CAD build for the part. Positions are in the model's coordinates, mm. Face numbers are marked on the shaded views. A direction names the side the tool comes from. Round coordinates to 2 decimals unless told otherwise and drop trailing zeros. Order: outer loops, then holes, each group sorted by start corner. A loop starts at its lowest first (then second) coordinate and runs counter-clockwise, first axis right, second up. Notation, with made-up numbers: (53, 18.5) -> (70, 18.5) arc R10 ccw to (70, 34.5) -> close; hole circle Ø10 at (37, 72.25). An arc over 180 degrees is marked (long way). Return JSON: item names as keys, results as strings. Group by question number.
Q1. Cut at D-D (y = 770). Write the cut outline in (x, z) (3 decimals), then the cut area to 3 significant figures.
Q2. Which spindle directions (+Z, -Z, +X, -X, +Y, -Y) get a long thin tool onto all of the face, cutting with end or side? Do the marked faces 1, 2, 3, 4 and 5. Say none if no direction does.
Q3. Cut at B-B (x = -514). Write the cut outline in (y, z) (3 decimals), then the cut area to 3 significant figures.
Q4. Cut at C-C (z = -218). Write the cut outline in (x, y) (1 decimal).
Q5. Cut at A-A (y = 467.5). Write the cut outline in (x, z) (3 decimals).
Q6. Probe line 1 along Z through (x, y) = (-279, 176.5) (3 decimals); line 2 along X through (y, z) = (471.5, -194); line 3 along Y through (x, z) = (-51.5, -27.5) (3 decimals). List the from-to ranges inside material, lowest first.
Q7. Mould opens along Z. For the marked faces 6, 7 and 8 say: +Z half, -Z half, draft (parallel to the pull), parting line (faces both ways), or undercut.
Q8. Flat gauge pins, fed straight in: pin 1 (4 mm diameter, centred on y = 330.5, z = -180, fed in from +X); pin 2 (3 mm diameter, centred on x = -550, z = -343, fed in from -Y); pin 3 (1.5 mm diameter, centred on y = 551, z = -132, fed in from +X). Where does each tip first touch, or does it go through?
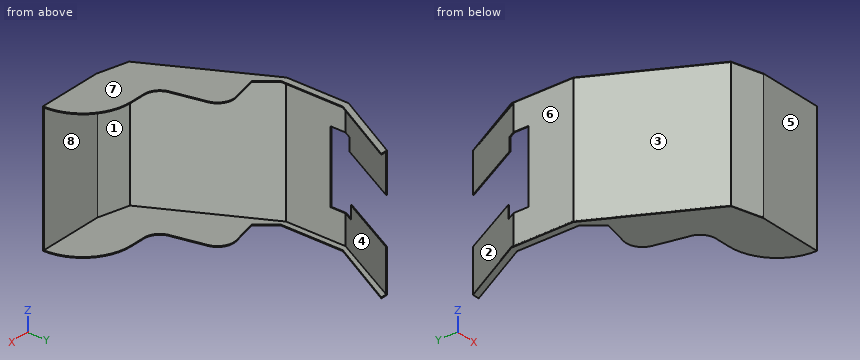
Autodesk Inventor part; units mm, degrees
ref_plane "YZ Plane" through (0, 0, 0) normal (1, 0, 0) x (0, 1, 0)
ref_plane "XZ Plane" through (0, 0, 0) normal (0, 1, 0) x (-1, 0, 0)
sketch "Sketch1" plane through (0, 0, 0) normal (0, 0, 1) x (1, 0, 0)
  line L0 (0, 0) -> (-241.3, 0)
  line L1 (-352.8762, 28.575) -> (-241.3, 0)
  line L2 (-568.379, 431.8) -> (-352.8762, 28.575)
  arc A0 (-1.9317, 0) -> (-179.7317, 177.8) centre (-179.7317, 0) ccw
  arc A1 (-321.8515, 344.496) -> (-394.4455, 390.1126) centre (-380.6333, 331.522) ccw
  line L3 (-179.7317, 177.8) -> (-238.6526, 177.8)
  line L4 (-321.8515, 344.496) -> (-296.6352, 230.2477)
  arc A2 (-296.6352, 230.2477) -> (-238.6526, 177.8) centre (-238.6526, 236.0747) ccw
  line L5 (-490.4406, 367.4826) -> (-394.4455, 390.1126)
  line L6 (-568.379, 431.8) -> (-568.379, 660.4)
  line L7 (-542.979, 660.4) -> (-542.979, 431.8)
  line L8 (-542.979, 431.8) -> (-490.4406, 367.4826)
  line L9 (-431.7117, 914.4) -> (-568.379, 660.4)
  line L10 (-406.3016, 914.4) -> (-542.979, 660.4)
  line L11 (-406.3016, 914.4) -> (-431.7117, 914.4)
sketch "Sketch4" plane through (0, 0, 0) normal (0, 0, 1) x (1, 0, 0)
  line L0 (-0.2535, 0) -> (-241.5535, 0)
  line L1 (-353.1324, 28.571) -> (-241.5535, 0)
  line L2 (-568.6352, 431.796) -> (-353.1324, 28.571)
  line L3 (-568.6352, 431.796) -> (-568.6352, 652.411)
  line L4 (-565.4602, 651.6325) -> (-565.4602, 432.585)
  line L5 (-431.9451, 914.3967) -> (-568.6352, 652.411)
  line L6 (-428.3639, 914.3967) -> (-565.4602, 651.6325)
  line L7 (-428.3639, 914.3967) -> (-431.9451, 914.3967)
  line L8 (-2.1852, 0) -> (-2.1852, 3.175)
  line L9 (-241.5535, 0) -> (-228.8535, 0)
  line L10 (-228.8535, 0) -> (-228.8535, 3.175)
  line L11 (-2.1852, 3.175) -> (-228.8535, 3.175)
  line L12 (-241.5535, 0) -> (-241.5535, 3.175)
  line L13 (-353.1324, 28.571) -> (-353.1324, 31.746)
  line L14 (-353.1324, 31.746) -> (-241.5535, 3.175)
  line L15 (-353.1324, 31.746) -> (-565.4602, 432.585)
  line L16 (-241.5535, 3.175) -> (-228.8535, 3.175)
  line L17 (-565.4602, 432.585) -> (-568.2578, 431.0898)
  line L18 (-565.4602, 651.6325) -> (-568.6352, 652.411)
  point P0 (0, 0)
  dimension "d63" = 3.175
  dimension "d64" = 12.7
  dimension "d65" = 3.175
  dimension "d66" = 3.175
  dimension "d68" = 3.175
  dimension "d90" = 3.175
  dimension "d92" = 3.175
  dimension "d93" = 3.175
  dimension "d96" = 0
  dimension "d97" = 0
extrude "Extrusion1" add sketch "Sketch4" against normal blind 469.9
extrude "Extrusion2" add sketch "Sketch1" along normal blind 3.175
ref_plane "Work Plane3" through (0, 0, -469.9) normal (0, 0, 1) x (1, 0, 0)
sketch "Sketch5" plane through (0, 0, 0) normal (0, 0, 1) x (1, 0, 0)
  line L0 (0, 0) -> (-241.3, 0)
  line L1 (-352.8762, 28.575) -> (-241.3, 0)
  line L2 (-568.379, 431.8) -> (-352.8762, 28.575)
  arc A0 (-1.9317, 0) -> (-179.7317, 177.8) centre (-179.7317, 0) ccw
  arc A1 (-321.8515, 344.496) -> (-394.4455, 390.1126) centre (-380.6333, 331.522) ccw
  line L3 (-179.7317, 177.8) -> (-238.6526, 177.8)
  line L4 (-321.8515, 344.496) -> (-296.6352, 230.2477)
  arc A2 (-296.6352, 230.2477) -> (-238.6526, 177.8) centre (-238.6526, 236.0747) ccw
  line L5 (-490.4406, 367.4826) -> (-394.4455, 390.1126)
  line L6 (-568.379, 431.8) -> (-568.379, 660.4)
  line L7 (-542.979, 660.4) -> (-542.979, 431.8)
  line L8 (-542.979, 431.8) -> (-490.4406, 367.4826)
  line L9 (-431.7117, 914.4) -> (-568.379, 660.4)
  line L10 (-406.3016, 914.4) -> (-542.979, 660.4)
  line L11 (-406.3016, 914.4) -> (-431.7117, 914.4)
sketch "Sketch6" plane through (0, 0, -469.9) normal (0, 0, 1) x (1, 0, 0)
  point P0 (0, 0)
sketch "Sketch7" plane through (0, 0, -469.9) normal (0, 0, 1) x (1, 0, 0)
  line L0 (0, 0) -> (-241.3, 0)
  line L1 (-352.8762, 28.575) -> (-241.3, 0)
  line L2 (-568.379, 431.8) -> (-352.8762, 28.575)
  arc A0 (-1.9317, 0) -> (-179.7317, 177.8) centre (-179.7317, 0) ccw
  arc A1 (-321.8515, 344.496) -> (-394.4455, 390.1126) centre (-380.6333, 331.522) ccw
  line L3 (-179.7317, 177.8) -> (-238.6526, 177.8)
  line L4 (-321.8515, 344.496) -> (-296.6352, 230.2477)
  arc A2 (-296.6352, 230.2477) -> (-238.6526, 177.8) centre (-238.6526, 236.0747) ccw
  line L5 (-490.4406, 367.4826) -> (-394.4455, 390.1126)
  line L6 (-568.379, 431.8) -> (-568.379, 660.4)
  line L7 (-542.979, 660.4) -> (-542.979, 431.8)
  line L8 (-542.979, 431.8) -> (-490.4406, 367.4826)
  line L9 (-431.7117, 914.4) -> (-568.379, 660.4)
  line L10 (-406.3016, 914.4) -> (-542.979, 660.4)
  line L11 (-406.3016, 914.4) -> (-431.7117, 914.4)
extrude "Extrusion3" add sketch "Sketch7" against normal blind 3.175
sketch "Sketch8" plane through (0, 0, 0) normal (1, 0, 0) x (0, 1, 0)
  line L0 (0, 0) -> (0, -228.6)
  line L1 (0, -473.075) -> (0, 3.175)
  line L2 (0, -228.6) -> (596.9, -228.6)
  line L3 (651.6325, -473.075) -> (651.6325, 3.175)
  line L4 (596.9, -228.6) -> (596.9, -95.25)
  line L5 (432.585, 0) -> (432.585, -469.9)
  line L6 (596.9, -228.6) -> (596.9, -361.95)
  line L7 (596.9, -361.95) -> (1104.9, -361.95)
  line L8 (1104.9, -361.95) -> (1104.9, -95.25)
  line L9 (1104.9, -95.25) -> (596.9, -95.25)
  line L10 (596.9, -95.25) -> (651.6325, -95.25)
  line L11 (651.6325, -95.25) -> (677.0325, -95.25)
  line L12 (677.0325, -95.25) -> (677.0325, -142.875)
  line L13 (677.0325, -142.875) -> (1104.9, -142.875)
  line L14 (651.6325, -361.95) -> (685.8, -361.95)
  line L15 (685.8, -361.95) -> (685.8, -314.325)
  line L16 (685.8, -314.325) -> (1104.9, -314.325)
  point P0 (660.4, -473.075)
  point P1 (660.4, 3.175)
  point P2 (431.8, 0)
  point P3 (431.8, -469.9)
  point P4 (432.585, -469.9)
  dimension "d77" = 228.6
  dimension "d78" = 596.9
  dimension "d80" = 133.35
  dimension "d81" = 133.35
  dimension "d82" = 508
  dimension "d83" = 266.7
  dimension "d84" = 25.4
  dimension "d85" = 47.625
  dimension "d86" = 47.625
extrude "Extrusion4" cut sketch "Sketch8" against normal blind 914.4 contours L7 L6 L4 L9 L3 | L3 L9 L12 L13 L8 L16 L15 L7
equation "\"SeatBottomDepth\" = 241.3"
equation "\"SeatFrontBottomWidth\" = 469.9"
equation "\"SeatFrontSidesWidth\" = 520.7"
equation "\"SeatBackInnerWidth\" = 304.8"
equation "\"SeatBackOuterWidth\" = 482.6"
equation "\"SeatBackLength\" = 457.2"
properties part number "Seat3DSketch"
Solution:
{
 "1": {"outline": "(-509.408, -473.075) -> (-484.003, -473.075) -> (-484.003, -469.9) -> (-503.702, -469.9) -> (-503.702, -314.325) -> (-507.284, -314.325) -> (-507.284, -469.9) -> (-509.408, -469.9) -> close; (-509.408, 0) -> (-507.284, 0) -> (-507.284, -142.875) -> (-503.702, -142.875) -> (-503.702, 0) -> (-484.003, 0) -> (-484.003, 3.175) -> (-509.408, 3.175) -> close", "area": "1,230 mm²"},
 "2": {"face 1": "+X, +Y", "face 2": "-X, +Y", "face 3": "+Z, -Z, -X, -Y", "face 4": "+X", "face 5": "+Z, -Z, +X, -X, -Y"},
 "3": {"outline": "(329.569, -469.9) -> (330.052, -469.9) -> (330.052, -473.075) -> (396.324, -473.075) -> (396.324, -469.9) -> (335.437, -469.9) -> (335.437, 0) -> (396.324, 0) -> (396.324, 3.175) -> (330.052, 3.175) -> (330.052, 0) -> (329.569, 0) -> close; (714.254, -473.075) -> (761.465, -473.075) -> (761.465, -469.9) -> (757.127, -469.9) -> (757.127, -314.325) -> (750.263, -314.325) -> (750.263, -469.9) -> (714.254, -469.9) -> close; (714.254, 0) -> (750.263, 0) -> (750.263, -142.875) -> (757.127, -142.875) -> (757.127, 0) -> (761.465, 0) -> (761.465, 3.175) -> (714.254, 3.175) -> close", "area": "5,530 mm²"},
 "4": {"outline": "(-568.6, 431.8) -> (-353.1, 28.6) -> (-241.6, 0) -> (-2.2, 0) -> (-2.2, 3.2) -> (-241.6, 3.2) -> (-353.1, 31.7) -> (-565.5, 432.6) -> (-565.5, 596.9) -> (-568.6, 596.9) -> close"},
 "5": {"outline": "(-568.635, -469.9) -> (-568.379, -469.9) -> (-568.379, -473.075) -> (-542.979, -473.075) -> (-542.979, -469.9) -> (-565.46, -469.9) -> (-565.46, 0) -> (-542.979, 0) -> (-542.979, 3.175) -> (-568.379, 3.175) -> (-568.379, 0) -> (-568.635, 0) -> close"},
 "6": {"line 1": "z = -473.075 to -469.9, 0 to 3.175", "line 2": "x = -568.64 to -565.46", "line 3": "y = 0 to 3.175"},
 "7": {"face 6": "draft", "face 7": "+Z half", "face 8": "undercut"},
 "8": {"pin 1": "stops at x = -510.33", "pin 2": "stops at y = 394.12", "pin 3": "stops at x = -565.46"}
}
